Can you work these out from the model? Positions are in its coordinate system, mm. Give positions to 0.01 mm unless a question says otherwise; leave off trailing zeros. One line per item, written item: value. Start each with the question number.
from build123d import *

# Parameters (mm, degrees)
SKETCH1_W                                         = 279.4
SKETCH1_H                                         = 57.15
SKETCH1_R                                         = 2.15265
SKETCH1_W_2                                       = 6.604
SKETCH1_H_2                                       = 6.35
BOSS_EXTRUDE1_DEPTH                               = 6.604
CSK_FOR_8_FLAT_HEAD_SOCKET_CAP_SCREW1_D           = 4.3053
CSK_FOR_8_FLAT_HEAD_SOCKET_CAP_SCREW1_CSINK_D     = 9.1186
CSK_FOR_8_FLAT_HEAD_SOCKET_CAP_SCREW1_CSINK_ANGLE = 82
F_8_32_TAPPED_HOLE1_D                             = 3.4544
F_8_32_TAPPED_HOLE1_DEPTH                         = 10.7188
F_8_32_TAPPED_HOLE1_TIP                           = 1.037806461


with BuildPart() as part:
    # Sketch1 → Boss-Extrude1 (new body)
    with BuildSketch(Plane(origin=(0, 0, 0), x_dir=(0, 0, -1), z_dir=(1, 0, 0))):
        Rectangle(SKETCH1_W, SKETCH1_H)
        with Locations((-133.35, 9.525)):
            Circle(SKETCH1_R, mode=Mode.SUBTRACT)
        with Locations((-133.35, -9.525)):
            Circle(SKETCH1_R, mode=Mode.SUBTRACT)
        with Locations((133.35, 9.525)):
            Circle(SKETCH1_R, mode=Mode.SUBTRACT)
        with Locations((133.35, -9.525)):
            Circle(SKETCH1_R, mode=Mode.SUBTRACT)
        with Locations((-133.35, 0)):
            Rectangle(SKETCH1_W_2, SKETCH1_H_2, mode=Mode.SUBTRACT)
        with Locations((-133.35, 19.05)):
            Rectangle(SKETCH1_W_2, SKETCH1_H_2, mode=Mode.SUBTRACT)
        with Locations((-133.35, -19.05)):
            Rectangle(SKETCH1_W_2, SKETCH1_H_2, mode=Mode.SUBTRACT)
        with Locations((133.35, 0)):
            Rectangle(SKETCH1_W_2, SKETCH1_H_2, mode=Mode.SUBTRACT)
        with Locations((133.35, 19.05)):
            Rectangle(SKETCH1_W_2, SKETCH1_H_2, mode=Mode.SUBTRACT)
        with Locations((133.35, -19.05)):
            Rectangle(SKETCH1_W_2, SKETCH1_H_2, mode=Mode.SUBTRACT)
    extrude(amount=BOSS_EXTRUDE1_DEPTH)

    # CSK for #8 Flat Head Socket Cap Screw1 (through all)
    with Locations(Plane(origin=(6.604, 0, 0), x_dir=(0, 0, -1), z_dir=(1, 0, 0))):
        with Locations((-133.35, 9.525), (-133.35, -9.525), (133.35, 9.525), (133.35, -9.525)):
            CounterSinkHole(CSK_FOR_8_FLAT_HEAD_SOCKET_CAP_SCREW1_D / 2, CSK_FOR_8_FLAT_HEAD_SOCKET_CAP_SCREW1_CSINK_D / 2, counter_sink_angle=CSK_FOR_8_FLAT_HEAD_SOCKET_CAP_SCREW1_CSINK_ANGLE)

    # #8-32 Tapped Hole1
    with Locations(Plane(origin=(6.604, 0, 0), x_dir=(0, 0, -1), z_dir=(1, 0, 0))):
        with Locations((-88.9, 0), (0, 0)):
            Hole(F_8_32_TAPPED_HOLE1_D / 2, depth=F_8_32_TAPPED_HOLE1_DEPTH)
            with Locations((0, 0, -(F_8_32_TAPPED_HOLE1_DEPTH + F_8_32_TAPPED_HOLE1_TIP / 2))):  # 118° drill point
                Cone(0, F_8_32_TAPPED_HOLE1_D / 2, F_8_32_TAPPED_HOLE1_TIP, mode=Mode.SUBTRACT)


solid = part.part
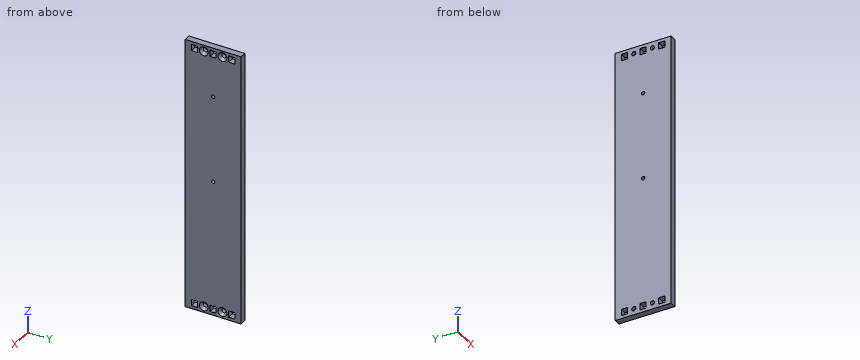
Q1. I need wall thicknesses on line 1 along Y through (x, z) = (2.4, -133.35) (3 decimals); line 2 along Z through (x, y) = (5.5, 16.5); line 3 along Y through (x, z) = (4.75, 0) (3 decimals). Which ranges of each line are inside material? Lowest first, please.
Q2. If we section it at A-A, the plane x = 1: Give the number of separate pieces and of enclosed holes in the cut face, plus the area to 3 significant figures.
Q3. For P1, Ø5, axis at y = -9.525, z = -133.35, coming from the +X side; P2, Ø7, axis at y = 9.525, z = 133.35, coming from the +X side, each with a flat end and sliding along its axis, tell me the tip position at first contact or that it passes through.
Response:
1. line 1: -28.575 to -22.225, -15.875 to -11.678, -7.372 to -3.175, 3.175 to 7.372, 11.678 to 15.875, 22.225 to 28.575
1. line 2: -139.7 to -136.65, -130.05 to 130.05, 136.65 to 139.7
1. line 3: -28.575 to -1.727, 1.727 to 28.575
2. separate pieces: 1
2. enclosed holes: 12
2. area: 15,600 mm^2
3. P1: x = 4.24
3. P2: x = 5.39
